Source: CAD feature listing. Evaluate the final solid. Frame: model axes, mm. Face numbers are marked on the shaded views. A direction names the side the tool comes from. Round coordinates to 2 decimals unless told otherwise and drop trailing zeros. Loops run counter-clockwise (first coordinate to the right, second up) from the corner with the lowest first, then second, coordinate; pieces in that order, holes last. Notation, with made-up numbers: M 20.5,-23.5 L 31.5,-23.5 A11 ccw 31.5,-4.5 Z; hole C 75,59 d5. An arc over 180 degrees is marked long. One line per item, written item: value.
from build123d import *

# Parameters (mm, degrees)
SKETCH_1_R          = 1.25
EXTRUDE_1_DEPTH     = 24
SKETCH_2_R          = 27.5
CUT_EXTRUDE_1_DEPTH = 21
FILLET_1_R          = 3
SKETCH_3_R          = 1.25
CUT_EXTRUDE_2_DEPTH = 31.645010485
CHAMFER_2_SIZE      = 1
CUT_EXTRUDE_3_DEPTH = 29.75
SKETCH_5_R          = 1.95
CUT_EXTRUDE_4_DEPTH = 2
SKETCH_6_R          = 1.95
CUT_EXTRUDE_5_DEPTH = 1


with BuildPart() as part:
    # Эскиз1 → Бобышка-Вытянуть1 (new body)
    with BuildSketch(Plane(origin=(0, 0, 0), x_dir=(1, 0, 0), z_dir=(0, 1, 0))):
        with BuildLine():
            Line((32.75, 13), (16.492422502, 13))
            ThreePointArc((16.492422502, 13), (19.841129914, 6.879648517), (21, 0))
            ThreePointArc((21, 0), (19.841129914, -6.879648517), (16.492422502, -13))
            Line((16.492422502, -13), (32.75, -13))
            Line((32.75, -13), (32.75, 13))
        make_face()
        with Locations(Location((23.685438565, -8, 0), (0, 0, 270))):
            Circle(SKETCH_1_R, mode=Mode.SUBTRACT)
        with Locations(Location((23.685438565, 8, 0), (0, 0, 270))):
            Circle(SKETCH_1_R, mode=Mode.SUBTRACT)
    extrude(amount=EXTRUDE_1_DEPTH)

    # Эскиз2 → Вырез-Вытянуть1 (cut)
    with BuildSketch(Plane(origin=(0, 24, 0), x_dir=(1, 0, 0), z_dir=(0, 1, 0))):
        Circle(SKETCH_2_R)
    extrude(amount=-CUT_EXTRUDE_1_DEPTH, mode=Mode.SUBTRACT)

    # Скругление1
    fillet_1_edges = [part.edges().sort_by_distance(p)[0] for p in [
        (16.492422502, 1.5, -13),
        (16.492422502, 1.5, 13),
        (24.233241632, 13.5, 13),
        (24.233241632, 13.5, -13),
    ]]
    fillet(fillet_1_edges, radius=FILLET_1_R)

    # Эскиз3 → Вырез-Вытянуть2 (cut, through all)
    with BuildSketch(Plane(origin=(32.75, 0, 0), x_dir=(0, 0, -1), z_dir=(1, 0, 0))):
        with Locations((0, 10.5)):
            Circle(SKETCH_3_R)
        with Locations((-10, 16)):
            Circle(SKETCH_3_R)
        with Locations((-10, 8)):
            Circle(SKETCH_3_R)
        with Locations(Location((10, 8, 0), (0, 0, 141.895375662))):
            Circle(SKETCH_3_R)
        with Locations(Location((10, 16, 0), (0, 0, 141.895375662))):
            Circle(SKETCH_3_R)
    extrude(amount=-CUT_EXTRUDE_2_DEPTH, mode=Mode.SUBTRACT)

    # Фаска2
    chamfer_2_edges = [part.edges().sort_by_distance(p)[0] for p in [
        (30.782029534, 24, 13),
        (27.283712115, 0, 13),
        (27.5, 24, 0),
        (30.782029534, 24, -13),
        (26.369593925, 24, -11.73913489),
        (26.369593925, 24, 11.73913489),
        (27.283712115, 0, -13),
        (21, 0, 0),
        (19.292547995, 0, 11.620185175),
        (19.292547995, 0, -11.620185175),
    ]]
    chamfer(chamfer_2_edges, length=CHAMFER_2_SIZE)

    # Эскиз4 → Вырез-Вытянуть3 (cut)
    with BuildSketch(Plane(origin=(0, 0, 0), x_dir=(0, 0, -1), z_dir=(1, 0, 0))):
        Polygon((-7.85, 14.758696921), (-7.85, 17.241303079), (-10, 18.482606158), (-12.15, 17.241303079), (-12.15, 14.758696921), (-10, 13.517393842), align=None)
        Polygon((-10, 10.482606158), (-7.85, 9.241303079), (-7.85, 6.758696921), (-10, 5.517393842), (-12.15, 6.758696921), (-12.15, 9.241303079), align=None)
        Polygon((7.85, 9.241303079), (7.85, 6.758696921), (10, 5.517393842), (12.15, 6.758696921), (12.15, 9.241303079), (10, 10.482606158), align=None)
        Polygon((10, 13.517393842), (7.85, 14.758696921), (7.85, 17.241303079), (10, 18.482606158), (12.15, 17.241303079), (12.15, 14.758696921), align=None)
    extrude(amount=CUT_EXTRUDE_3_DEPTH, mode=Mode.SUBTRACT)

    # Эскиз5 → Вырез-Вытянуть4 (cut)
    with BuildSketch(Plane(origin=(32.75, 0, 0), x_dir=(0, 0, -1), z_dir=(1, 0, 0))):
        with Locations((0, 10.5)):
            Circle(SKETCH_5_R)
    extrude(amount=-CUT_EXTRUDE_4_DEPTH, mode=Mode.SUBTRACT)

    # Эскиз6 → Вырез-Вытянуть5 (cut)
    with BuildSketch(Plane.XZ):
        with Locations(Location((23.685438565, 8, 0), (0, 0, 270))):
            Circle(SKETCH_6_R)
        with Locations(Location((23.685438565, -8, 0), (0, 0, 270))):
            Circle(SKETCH_6_R)
    extrude(amount=-CUT_EXTRUDE_5_DEPTH, mode=Mode.SUBTRACT)


solid = part.part
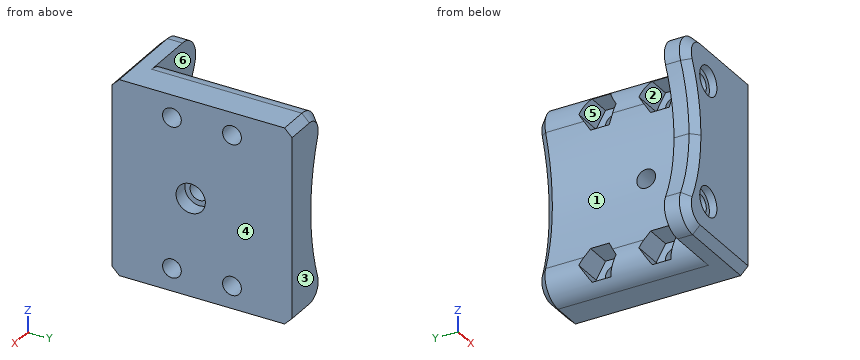
1. Reachability of the marked faces 1, 2 and 3 from +Z, -Z, +X, -X, +Y, -Y: full face, straight path, thin tool, end or side. Return the list, or none.
Report:
face 1: -X, +Y
face 2: -X
face 3: +Z, -Z, +X, -X, +Y
2. Ray query, line 1 (Y direction, x = 30.85, z = -10); line 2 (Y direction, x = 27.75, z = 9); line 3 (Y direction, x = 32.2, z = 0). Return the intervals inside material, ascending. Write a range as [from, to].
Report:
line 1: y = [0, 6.75], [9.25, 14.75], [17.25, 24]
line 2: y = [0, 6.09], [9.91, 14.09], [17.91, 24]
line 3: y = [0, 8.55], [12.45, 24]
3. Section query A-A (y = 8). Return the cut outline in (x, z).
Report:
outline: M 26.36,-7.85 L 29.75,-7.85 L 29.75,-8.75 L 32.75,-8.75 L 32.75,8.75 L 29.75,8.75 L 29.75,7.85 L 26.36,7.85 A27.5 cw Z; M 26.72,-12.15 A3 ccw 28.81,-13 L 32.75,-13 L 32.75,-11.25 L 29.75,-11.25 L 29.75,-12.15 Z; M 26.72,12.15 L 29.75,12.15 L 29.75,11.25 L 32.75,11.25 L 32.75,13 L 28.81,13 A3 ccw Z
4. Pin query (flat end, axial travel): pin 1 (1.5 mm diameter, centred on y = 8, z = 10, fed in from -X); pin 2 (5 mm diameter, centred on x = 21.5, z = -3, fed in from -Y); pin 3 (4 mm diameter, centred on y = 4, z = 8, fed in from -X); pin 4 (3 mm diameter, centred on y = 16, z = 10, fed in from -X). Return the tip coordinate at first contact, or that it passes through.
Report:
pin 1: passes through
pin 2: stops at y = 0
pin 3: stops at x = 18.83
pin 4: stops at x = 29.75
5. Section query B-B (y = 4.25). Return the cut outline in (x, z), and give its area (3 significant figures).
Report:
outline: M 25.98,-9.02 A3 ccw 28.81,-13 L 32.75,-13 L 32.75,13 L 28.81,13 A3 ccw 25.98,9.02 A27.5 cw Z
area: 155 mm2
6. Pull-direction query (Y, two-part tool) for the marked faces 4, 5 and 6; classes: released by +Y, released by -Y, zero draft, split by the parting line, or undercut.
Report:
face 4: zero draft
face 5: undercut
face 6: released by +Y
